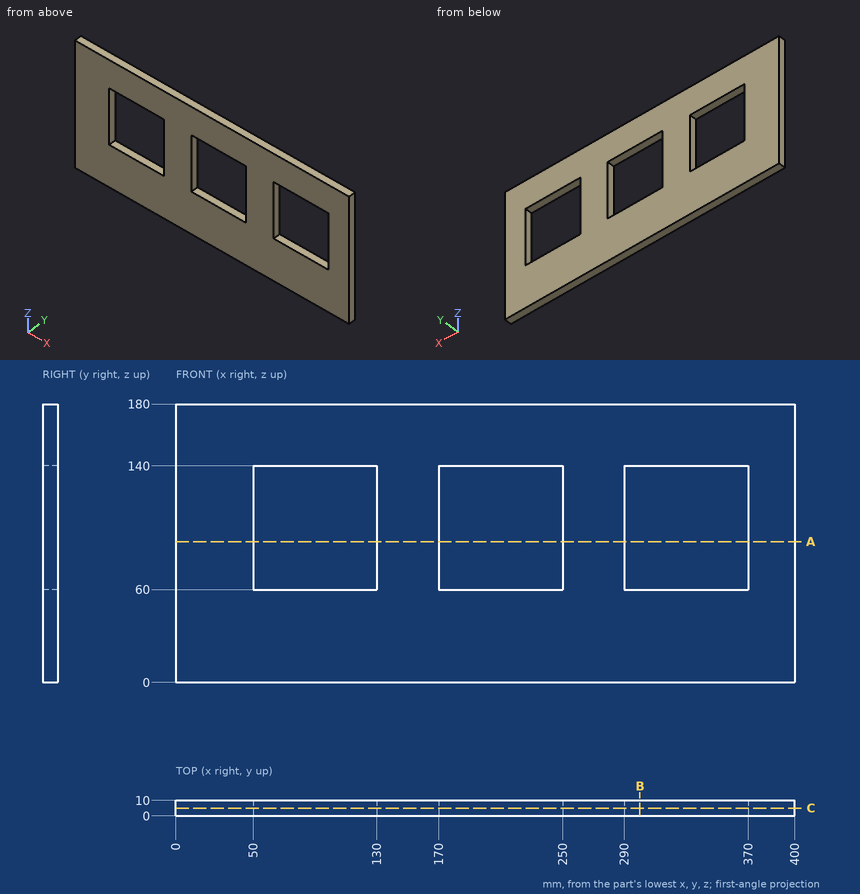
Here's the drawing with two shaded views (mm, measured from the low corner). I have some questions. Give positions to 0.01 mm unless a question says otherwise; leave off trailing zeros. Order: outer loops, then holes, each group sorted by start corner. A loop starts at its lowest first (then second) coordinate and runs counter-clockwise, first axis right, second up. Notation, with made-up numbers: (34, 19.5) - (50, 19.5) arc R22 cw to (50, 41.5) - close; hole circle Ø6 at (86, -37). An arc over 180 degrees is marked (long way). Use a Markdown table: item, result. Add a question column.
Q1. Please list where these lines run through material, in increasing order: line 1 along X through (y, z) = (2.5, 101.5); line 2 along Z through (x, y) = (241, 0.5).
Q2. If we section it at B-B on x = 300: Write out the boundary of the cut face in (y, z).
Q3. If we section it at A-A on z = 91: Write out the boundary of the cut face in (x, y), plus the area to 3 significant figures.
Q4. If we section it at C-C on y = 5: Write out the boundary of the cut face in (x, z).
Q5. I'm going to push a flat-ended pin straight in: pin 1 (5 mm diameter, centred on y = 6.5, z = 92.5, fed in from -X). Where does the tip first touch, or does it pass through?
Answers follow:
| question | item | result |
|---|---|---|
| 1 | line 1 | x = 0 to 50, 130 to 170, 250 to 290, 370 to 400 |
| 1 | line 2 | z = 0 to 60, 140 to 180 |
| 2 | outline | (0, 0) - (10, 0) - (10, 60) - (0, 60) - close; (0, 140) - (10, 140) - (10, 180) - (0, 180) - close |
| 3 | outline | (0, 0) - (50, 0) - (50, 10) - (0, 10) - close; (130, 0) - (170, 0) - (170, 10) - (130, 10) - close; (250, 0) - (290, 0) - (290, 10) - (250, 10) - close; (370, 0) - (400, 0) - (400, 10) - (370, 10) - close |
| 3 | area | 1,600 mm^2 |
| 4 | outline | (0, 0) - (400, 0) - (400, 180) - (0, 180) - close; hole (50, 60) - (130, 60) - (130, 140) - (50, 140) - close; hole (170, 60) - (250, 60) - (250, 140) - (170, 140) - close; hole (290, 60) - (370, 60) - (370, 140) - (290, 140) - close |
| 5 | pin 1 | stops at x = 0 |
